Can you work these out from the model? Positions are in its coordinate system, mm. Face numbers are marked on the shaded views. Coordinates: 2 decimals unless noted, no trailing zeros. Loops run counter-clockwise (first coordinate to the right, second up) from the corner with the lowest first, then second, coordinate; pieces in that order, holes last. Notation, with made-up numbers: M 28.5,-30.75 L 65.5,-30.75 A15 cw 65.5,-1.75 Z; hole C 80.25,-24 d6. An arc over 180 degrees is marked long. Answer as a JSON object with one key per item and string values. Group by question number.
Item 1: Suppose I cut it at D-D (x = -17.25). Write out the boundary of the cut face in (y, z), then the cut area to 3 significant figures.
Item 2: If I drill on line 1 (Z direction, x = -2, y = 2.35); line 2 (X direction, y = 0.65, z = -2.8); line 3 (X direction, y = 1.5, z = -1.4), over which ranges is the centre line in solid material (lowest first)?
Item 3: Suppose I cut it at A-A (z = -2). Write out the boundary of the cut face in (x, y), then the cut area to 3 significant figures.
Item 4: Suppose I cut it at B-B (x = -2). Write out the boundary of the cut face in (y, z).
Item 5: We'd pull the mould along X, two halves only. Please class the marked faces 1, 2, 3 and 4: +X half, -X half, draft (parallel to the pull), parting line (faces both ways), or undercut.
Item 6: Suppose I cut it at C-C (y = 0.75). Write out the boundary of the cut face in (x, z).
Autodesk Inventor part; units mm, degrees
ref_plane "YZ Plane" through (0, 0, 0) normal (1, 0, 0) x (0, 1, 0)
ref_plane "XZ Plane" through (0, 0, 0) normal (0, 1, 0) x (-1, 0, 0)
ref_plane "XY Plane" through (0, 0, 0) normal (0, 0, 1) x (1, 0, 0)
sketch "Sketch1" plane through (0, 0, 0) normal (0, 1, 0) x (-1, 0, 0)
  line L0 (0, 0) -> (20, 0)
  line L1 (20, 0) -> (20, -4)
  line L2 (20, -4) -> (0, -4)
  line L3 (0, -4) -> (0, 0)
  line L4 (0, -2) -> (2, -2)
  line L5 (20, -2) -> (18, -2)
  circle A0 centre (18, -2) radius 1
  circle A1 centre (2, -2) radius 1
  dimension "d0" = 20
  dimension "d1" = 4
  dimension "d2" = 2
  dimension "d3" = 2
  dimension "d4" = 2
  dimension "d5" = 2
extrude "Extrusion1" add sketch "Sketch1" along normal blind 4
properties part number "parallel_bar_short_v1"
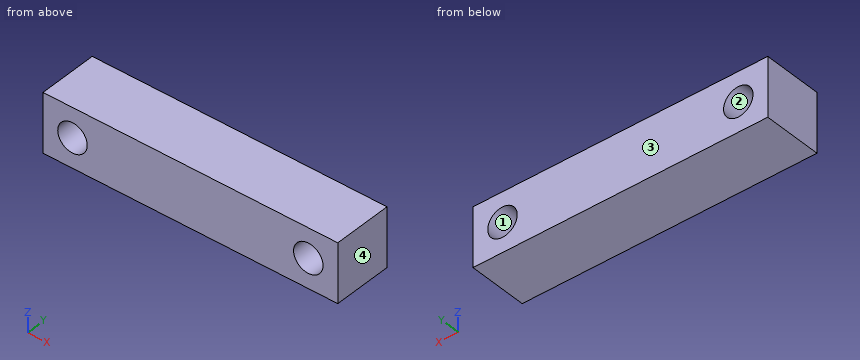
From the geometry:
{
 "1": {"outline": "M 0,-4 L 4,-4 L 4,-2.66 L 0,-2.66 Z; M 0,-1.34 L 4,-1.34 L 4,0 L 0,0 Z", "area": "10.7 mm2"},
 "2": {"line 1": "-4 to -3, -1 to 0", "line 2": "-20 to -18.6, -17.4 to -2.6, -1.4 to 0", "line 3": "-20 to -18.8, -17.2 to -2.8, -1.2 to 0"},
 "3": {"outline": "M -20,0 L -19,0 L -19,4 L -20,4 Z; M -17,0 L -3,0 L -3,4 L -17,4 Z; M -1,0 L 0,0 L 0,4 L -1,4 Z", "area": "64.0 mm2"},
 "4": {"outline": "M 0,-4 L 4,-4 L 4,-3 L 0,-3 Z; M 0,-1 L 4,-1 L 4,0 L 0,0 Z"},
 "5": {"face 1": "undercut", "face 2": "undercut", "face 3": "draft", "face 4": "+X half"},
 "6": {"outline": "M -20,-4 L 0,-4 L 0,0 L -20,0 Z; hole C -18,-2 d2; hole C -2,-2 d2"}
}
